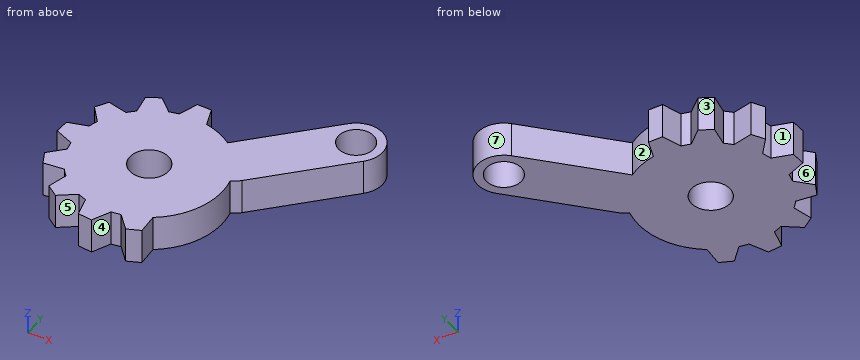
from build123d import *

# Parameters (mm, degrees)
CROQUIS1_R               = 5
SALIENTE_EXTRUIR5_DEPTH  = 10
MATRIZC4_COUNT           = 8
MATRIZC4_ANGLE           = 203
CROQUIS9_R               = 5
SALIENTE_EXTRUIR6_DEPTH  = 10
SALIENTE_EXTRUIR7_START  = -10
CROQUIS11_R              = 5
SALIENTE_EXTRUIR7_DEPTH  = 10
CORTAR_EXTRUIR2_DEPTH    = 10
SALIENTE_EXTRUIR9_DEPTH  = 10
CROQUIS15_R              = 6
CORTAR_EXTRUIR4_DEPTH    = 10
ESCALA1_SCALE            = 0.75
CROQUIS16_R              = 4.5
CROQUIS16_R_2            = 4.125
SALIENTE_EXTRUIR12_DEPTH = 7.5


with BuildPart() as part:
    # Croquis1 → Saliente-Extruir5 (new body)
    with BuildSketch(Plane.XY):
        with BuildLine():
            Line((-2, 25.706379875), (-3.901693271, 20.335460584))
            ThreePointArc((-3.901693271, 20.335460584), (0, -20.706379875), (3.901693271, 20.335460584))
            Line((3.901693271, 20.335460584), (2, 25.706379875))
            Line((2, 25.706379875), (-2, 25.706379875))
        make_face()
        Circle(CROQUIS1_R, mode=Mode.SUBTRACT)
    saliente_extruir5 = extrude(amount=SALIENTE_EXTRUIR5_DEPTH)

    # MatrizC4: Saliente-Extruir5 ×8 about axis
    matrizc4_axis = Axis((0, 0, 0), (0, 0, 1))
    for i in range(1, MATRIZC4_COUNT):
        add(saliente_extruir5.rotate(matrizc4_axis, i * MATRIZC4_ANGLE / (MATRIZC4_COUNT - 1)))

    # Croquis9 → Saliente-Extruir6 (add)
    with BuildSketch(Plane.XY.offset(10)):
        with BuildLine():
            Line((11.839442553, 16.776986757), (33.130186467, 38.526068093))
            ThreePointArc((33.130186467, 38.526068093), (43.736186818, 38.639012949), (43.849131674, 28.033012597))
            Line((43.849131674, 28.033012597), (22.558387761, 6.283931261))
            ThreePointArc((22.558387761, 6.283931261), (11.952387409, 6.170986405), (11.839442553, 16.776986757))
        make_face()
        with Locations((38.48965907, 33.279540345)):
            Circle(CROQUIS9_R, mode=Mode.SUBTRACT)
    extrude(amount=-SALIENTE_EXTRUIR6_DEPTH)

    # Croquis11 → Saliente-Extruir7 (add)
    with BuildSketch(Plane.XY.offset(10).offset(SALIENTE_EXTRUIR7_START)):
        Circle(CROQUIS11_R)
    extrude(amount=SALIENTE_EXTRUIR7_DEPTH)

    # Croquis12 → Cortar-Extruir2 (cut)
    with BuildSketch(Plane.XY.offset(10)):
        with BuildLine():
            ThreePointArc((-3.771236166, 4.666666667), (0, -6), (3.771236166, 4.666666667))
            ThreePointArc((3.771236166, 4.666666667), (0, 10), (-3.771236166, 4.666666667))
        make_face()
    extrude(amount=-CORTAR_EXTRUIR2_DEPTH, mode=Mode.SUBTRACT)

    # Croquis13 → Saliente-Extruir9 (add)
    with BuildSketch(Plane.XY.offset(10)):
        with BuildLine():
            ThreePointArc((3.771236166, 4.666666667), (0, 10), (-3.771236166, 4.666666667))
            ThreePointArc((-3.771236166, 4.666666667), (0, -6), (3.771236166, 4.666666667))
        make_face()
    extrude(amount=-SALIENTE_EXTRUIR9_DEPTH)

    # Croquis15 → Cortar-Extruir4 (cut)
    with BuildSketch(Plane.XY.offset(10)):
        Circle(CROQUIS15_R)
    extrude(amount=-CORTAR_EXTRUIR4_DEPTH, mode=Mode.SUBTRACT)


with BuildPart() as part_1:
    # Escala1: scaled about (5.677071508, 5.296040102, 5)
    add(part.part.scale(ESCALA1_SCALE).moved(Location((1.419267877, 1.324010026, 1.25))))

    # Croquis16 → Saliente-Extruir12 (add)
    with BuildSketch(Plane.XY.offset(8.75)):
        with Locations((1.419267877, 1.324010026)):
            Circle(CROQUIS16_R)
        with Locations((1.419267877, 1.324010026)):
            Circle(CROQUIS16_R_2, mode=Mode.SUBTRACT)
    extrude(amount=-SALIENTE_EXTRUIR12_DEPTH)


solid = part_1.part
Work out the finished part from the listing and answer in its coordinate system (mm). Face numbers are marked on the shaded views. A direction names the side the tool comes from. Give positions to 0.01 mm unless a question says otherwise; leave off trailing zeros. Order: outer loops, then holes, each group sorted by start corner. A loop starts at its lowest first (then second) coordinate and runs counter-clockwise, first axis right, second up. Notation, with made-up numbers: (-10, -34) - (-4, -34) arc R28 cw to (-4, -12) - close; hole circle Ø11 at (-23, -30.75). An arc over 180 degrees is marked (long way). Answer as CSV lines item,"result". Start each with the question number.
Q1. The part is cut by section C-C (x = 22). Write down the section's boundary in (y, z), then the cut area to 3 significant figures.
Q2. Find the intervals of material crossed by L1, parallel to X at y = 17, z = 7.5; L2, parallel to X at y = 1, z = 6; L3, parallel to X at y = 29, z = 6.5, in increasing order. Write a range as [from, to].
Q3. For the marked faces 1, 2, 3 and 4, determine the directions among +Z, -Z, +X, -X, +Y, -Y from which every point of the face is accessible in a straight line to the end or side of a thin tool.
Q4. The part is cut by section B-B (y = -6.5). Write down the section's boundary in (x, z).
Q5. The mould has two halves that part along X. Classify the marked faces 5, 6 and 7: +X half, -X half, draft (parallel to the pull), parting line (faces both ways), or undercut.
Q6. The part is cut by section A-A (z = 2.5). Give the number of separate pieces and of enclosed holes in the cut face, then the cut area to 3 significant figures.
Q7. Given pin 1 Ø1 at (y, z) = (22.5, 4.5) entering from +X; pin 2 Ø2.5 at (x, z) = (1, 5.5) entering from +Y, each flat-ended and moving along its own axis, determine where each tip first touches the part or whether it passes through.
Check result:
1,outline,"(9.78, 1.25) - (25.86, 1.25) - (25.86, 8.75) - (9.78, 8.75) - close"
1,area,"121 mm²"
2,L1,"x = [-9.16, -4.45], [-1.36, 4.2], [13.33, 29.07]"
2,L2,"x = [-17.9, -2.69], [5.53, 16.95]"
2,L3,"x = [25.07, 27.7], [32.87, 35.21]"
3,face 1,"+Z, -Z, -X"
3,face 2,"+Z, -Z, +Y"
3,face 3,"+Z, -Z, -X, +Y"
3,face 4,"+Z, -Z, -Y"
4,outline,"(-16.22, 1.25) - (14.83, 1.25) - (14.83, 8.75) - (-16.22, 8.75) - close"
5,face 5,"undercut"
5,face 6,"-X half"
5,face 7,"parting line"
6,separate pieces,"1"
6,enclosed holes,"2"
6,area,"1,100 mm²"
7,pin 1,"stops at x = 34.85"
7,pin 2,"stops at y = 20.6"
